Input: part model. Units: mm. Frame: model coordinates. A direction names the side the tool comes from. Coordinates: 2 decimals unless noted, no trailing zeros. Loops run counter-clockwise (first coordinate to the right, second up) from the corner with the lowest first, then second, coordinate; pieces in that order, holes last. Notation, with made-up numbers: (-27, -32) - (-16, -32) arc R31 ccw to (-16, -1) - close; hole circle Ø7 at (87.5, 18). An arc over 180 degrees is marked (long way). Use a Markdown table: item, result. Add a question column.
1. Section query A-A on z = 7.5. Return the cut outline in (x, y), then the cut area to 3 significant figures.
2. Ray query, L1, parallel to Y at x = -0.5, z = 3.5; L2, parallel to X at y = -4.5, z = 9.5; L3, parallel to Z at x = 11.2, y = 35. Return the intervals inside material, ascending. Write a range as [from, to].
3. Contact query for flat-ended pins moving along their axis: P1, Ø3, axis at y = -8, z = 10, coming from the -X side; P2, Ø5, axis at x = -23.5, z = 11, coming from the +Y side; P3, Ø7, axis at y = 35, z = 7.5, coming from the -X side; P4, Ø4, axis at x = -35, y = 0, coming from the -Z side. Output: stop coordinate, or through.
4. Section query B-B on y = -30. Return the cut outline in (x, z) (3 decimals).
5. Access query for faces 1 (the face through (-16, 38.3, 7.4)), 2 (the face through (-39, -3, 10)), 3 (the face through (26, 0, 8)), 4 (the face through (-10, 31.7, 7.4)). Directions: +Z, -Z, +X, -X, +Y, -Y. A direction counts if a zero-diameter tool reaches every point of the face in a straight line with its end or side. Return the directions, or none.
6. Draft query along Z for faces 5 (the face through (-32.8, 3.3, 5)), 6 (the face through (16, 31.7, 7.4)), 7 (the face through (-12.96, 32.47, 9.11)). Return one class per face: released by +Z, released by -Z, zero draft, split by the parting line, or undercut.
7. Section query D-D on x = -35. Return the cut outline in (y, z).
8. Section query C-C on z = 13. Return the cut outline in (x, y).
```python
from build123d import *

# Parameters (mm, degrees)
ESTRUSIONE_ESTRUSIONE1_DEPTH = 15
TAGLIO_ESTRUSIONE1_DEPTH     = 5
TAGLIO_ESTRUSIONE2_REACH     = 74.284
FORO_6_0_6_1_D               = 6


with BuildPart() as part:
    # Schizzo1 → Estrusione-Estrusione1 (new body)
    with BuildSketch(Plane.XY):
        with BuildLine():
            Line((-40, 30), (-16, 30))
            Line((-16, 30), (-16, 40))
            Line((-16, 40), (-10, 40))
            Line((-10, 40), (-10, 30))
            Line((-10, 30), (10, 30))
            Line((10, 30), (10, 40))
            Line((10, 40), (16, 40))
            Line((16, 40), (16, 30))
            Line((16, 30), (40, 30))
            ThreePointArc((40, 30), (0, -50), (-40, 30))
        make_face()
    extrude(amount=ESTRUSIONE_ESTRUSIONE1_DEPTH)

    # Schizzo2 → Taglio-Estrusione1 (cut)
    with BuildSketch(Plane.XY.offset(15)):
        with BuildLine():
            Line((16.05, 0), (16.05, -60))
            ThreePointArc((16.05, -60), (0, -76.05), (-16.05, -60))
            Line((-16.05, -60), (-16.05, 0))
            ThreePointArc((-16.05, 0), (0, 16.05), (16.05, 0))
        make_face()
    extrude(amount=-TAGLIO_ESTRUSIONE1_DEPTH, mode=Mode.SUBTRACT)

    # Schizzo3 → Taglio-Estrusione2 (cut, up to next)
    with BuildSketch(Plane.XY.offset(15), mode=Mode.PRIVATE) as taglio_estrusione2_sk1:
        with BuildLine():
            Line((29, 3), (41, 3))
            ThreePointArc((41, 3), (44, 0), (41, -3))
            Line((41, -3), (29, -3))
            ThreePointArc((29, -3), (26, 0), (29, 3))
        make_face()
    taglio_estrusione2_tool1 = extrude(taglio_estrusione2_sk1.sketch, amount=-TAGLIO_ESTRUSIONE2_REACH, mode=Mode.PRIVATE) & part.part
    add(taglio_estrusione2_tool1.solids().sort_by_distance((35, 0, 15))[0], mode=Mode.SUBTRACT)

    # Schizzo4 → Foro Ø24.0 (24)-1 (revolve, cut)
    with BuildSketch(Plane(origin=(0, 0, 10), x_dir=(0, -1, 0), z_dir=(1, 0, 0))):
        Polygon((0, 0), (0, 10.001), (12, 10.001), (12, 0.025), (12.025, 0), align=None)
    revolve(axis=Axis((0, 0, 16.35), (0, 0, -1)), mode=Mode.SUBTRACT)

    # Schizzo5 → Foro Ø10.0 (10)-1 (revolve, cut)
    with BuildSketch(Plane(origin=(0, -30, 10), x_dir=(0, -1, 0), z_dir=(1, 0, 0))):
        Polygon((0, 0), (0, 10.001), (5, 10.001), (5, 0.025), (5.025, 0), align=None)
    revolve(axis=Axis((0, -30, 16.35), (0, 0, -1)), mode=Mode.SUBTRACT)

    # Schizzo6 → Foro lamato per Bullone M5 a testa esagonale-1 (revolve, cut)
    with BuildSketch(Plane(origin=(-35, 0, 15), x_dir=(0, -1, 0), z_dir=(1, 0, 0))):
        Polygon((0, 0), (0, 15.001), (3.5, 15.001), (3.5, 10), (5, 10), (5, 0), align=None)
    revolve(axis=Axis((-35, 0, 21.35), (0, 0, -1)), mode=Mode.SUBTRACT)

    # Foro Ø6.0 (6)-1 (through all)
    with Locations(Plane(origin=(-16, 35, 7.5), x_dir=(0, 0, -1), z_dir=(-1, 0, 0))):
        with Locations((0, 0)):
            Hole(FORO_6_0_6_1_D / 2)


solid = part.part
```
Resolved:
| question | item | result |
|---|---|---|
| 1 | outline | (-40, 30) arc R50 ccw (long way) to (40, 30) - (16, 30) - (16, 32) - (10, 32) - (10, 30) - (-10, 30) - (-10, 32) - (-16, 32) - (-16, 30) - close; (-16, 38) - (-10, 38) - (-10, 40) - (-16, 40) - close; (10, 38) - (16, 38) - (16, 40) - (10, 40) - close; hole circle Ø10 at (-35, 0); hole circle Ø24 at (0, 0); hole circle Ø10 at (0, -30); hole (29, -3) - (41, -3) arc R3 ccw to (41, 3) - (29, 3) arc R3 ccw to start |
| 1 | area | 6,070 mm² |
| 2 | L1 | [-50, -34.97], [-25.03, -11.99], [11.99, 30] |
| 2 | L2 | [-49.8, -37.18], [-32.82, -11.12], [11.12, 49.8] |
| 2 | L3 | [0, 4.5], [10.5, 15] |
| 3 | P1 | x = -49.58 |
| 3 | P2 | y = 30 |
| 3 | P3 | x = -16 |
| 3 | P4 | through |
| 4 | outline | (-40, 0) - (-5, 0) - (-5, 9.975) - (-5.025, 10) - (-16.05, 10) - (-16.05, 15) - (-40, 15) - close; (5, 0) - (40, 0) - (40, 15) - (16.05, 15) - (16.05, 10) - (5.025, 10) - (5, 9.975) - close |
| 5 | face 1 | +Z, -Z, -X, +Y |
| 5 | face 2 | +Z |
| 5 | face 3 | +Z, -Z |
| 5 | face 4 | +Z, -Z, +Y |
| 6 | face 5 | released by +Z |
| 6 | face 6 | zero draft |
| 6 | face 7 | undercut |
| 7 | outline | (-35.71, 0) - (-3.5, 0) - (-3.5, 5) - (-5, 5) - (-5, 15) - (-35.71, 15) - close; (3.5, 0) - (30, 0) - (30, 15) - (5, 15) - (5, 5) - (3.5, 5) - close |
| 8 | outline | (-40, 30) arc R50 ccw to (-16.05, -47.35) - (-16.05, 0) arc R16.05 cw to (16.05, 0) - (16.05, -47.35) arc R50 ccw to (40, 30) - (16, 30) - (16, 40) - (10, 40) - (10, 30) - (-10, 30) - (-10, 40) - (-16, 40) - (-16, 30) - close; hole circle Ø10 at (-35, 0); hole (29, -3) - (41, -3) arc R3 ccw to (41, 3) - (29, 3) arc R3 ccw to start |
